Model file for the job. Use its own axes, mm. Face numbers are marked on the shaded views. Coordinates: 2 decimals unless noted, no trailing zeros. Loops run counter-clockwise (first coordinate to the right, second up) from the corner with the lowest first, then second, coordinate; pieces in that order, holes last.
from build123d import *

# Parameters (mm, degrees)
F0_R     = 69.85
F0_R_2   = 14.25
F1_DEPTH = 19.05
F0_R_3   = 1.5875
F2_DEPTH = 6.35
F3_R     = 6.35


with BuildPart() as f1:
    # F0 (on Top) → F1 (new body)
    with BuildSketch(Plane.XY):
        with Locations((91.948161, 93.335833)):
            Circle(F0_R)
        with Locations((91.948161, 93.335833)):
            Circle(F0_R_2, mode=Mode.SUBTRACT)
    extrude(amount=F1_DEPTH)

    # F0 (on Top) → F2 (join)
    with BuildSketch(Plane.XY):
        with Locations((91.948161, 93.335833)):
            Circle(F0_R_2)
        with Locations((91.948161, 86.210787)):
            Circle(F0_R_3, mode=Mode.SUBTRACT)
        with Locations((91.948161, 100.460879)):
            Circle(F0_R_3, mode=Mode.SUBTRACT)
    extrude(amount=F2_DEPTH)

    # F3
    f3_edges = [f1.edges().sort_by_distance(p)[0] for p in [
        (22.098161, 93.335833, 19.05),
    ]]
    fillet(f3_edges, radius=F3_R)


solid = f1.part
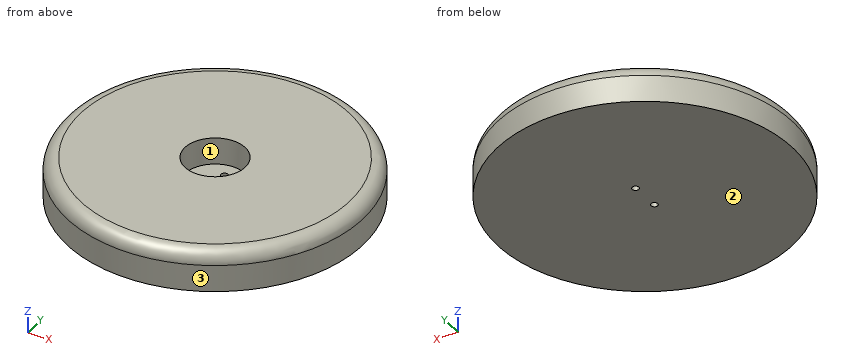
Q1. Flat gauge pins, fed straight in: P1, Ø4, axis at y = 80.5, z = 8, coming from the +X side; P2, Ø17, axis at x = 91.95, y = 93.34, coming from the -Z side; P3, Ø1.5, axis at x = 109.5, z = 9.5, coming from the -Y side; P4, Ø5, axis at x = 91.95, y = 86.21, coming from the +Z side. Where does each tip first touch, or does it go through?
Answers:
P1: stops at x = 160.95
P2: stops at z = 0
P3: stops at y = 25.54
P4: stops at z = 6.35
Q2. Mould opens along X. For the marked faces 1, 2 and 3 say: +X half, -X half, draft (parallel to the pull), parting line (faces both ways), or undercut.
Answers:
face 1: undercut
face 2: draft
face 3: parting line
Q3. Drill centre lines: line 1 (Y direction, x = 81.5, z = 13.25); line 2 (X direction, y = 85.5, z = 16.25); line 3 (Z direction, x = 91.5, y = 97.5). Where is each one in solid material? Low to high.
Answers:
line 1: y = 24.3 to 83.65, 103.03 to 162.38
line 2: x = 23.63 to 80.05, 103.85 to 160.27
line 3: z = 0 to 6.35
Q4. Slice it at A-A (z = 14.5). List the corners of the cut face in (x, y).
Answers:
outline: circle Ø139.18 at (91.95, 93.34); hole circle Ø28.5 at (91.95, 93.34)
